CAD build for the part. Positions are in the model's coordinates, mm. Coordinates: 2 decimals unless noted, no trailing zeros. Loops run counter-clockwise (first coordinate to the right, second up) from the corner with the lowest first, then second, coordinate; pieces in that order, holes last. Notation, with made-up numbers: (28.5, -11.75) -> (60.5, -11.75) arc R7 ccw to (60.5, -6.75) -> close; hole circle Ø5 at (9.25, 23.25). An arc over 180 degrees is marked (long way). Return JSON: item names as keys, results as strings. Group by question number.
(1) Saw through at A-A on x = 20.25. Write the cut outline in (y, z) (3 decimals).
(2) Flat gauge pins, fed straight in: pin 1 Ø10 at (x, z) = (17.5, 0.5) entering from -Y; pin 2 Ø2 at (x, z) = (3.5, -2.5) entering from -Y. Where does each tip first touch, or does it go through?
(3) Probe L1, parallel to Z at x = 19.75, y = 64 (3 decimals); L2, parallel to Z at x = 23.75, y = 63; L3, parallel to Y at x = 11, z = 11.5. List the from-to ranges inside material, lowest first.
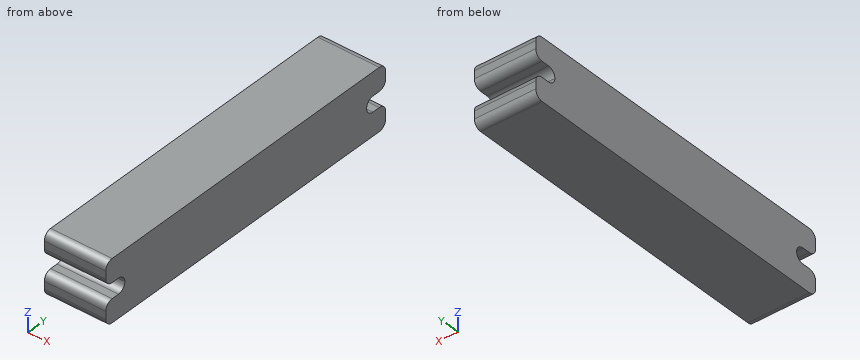
```python
from build123d import *

# Parameters (mm, degrees)
F1_DEPTH = 25.4


with BuildPart() as f1:
    # F0 (on Right) → F1 (new body)
    with BuildSketch(Plane.YZ):
        with BuildLine():
            Line((66.675, 12.7), (-66.675, 12.7))
            ThreePointArc((-66.675, 12.7), (-68.920064, 11.770064), (-69.85, 9.525))
            Line((-69.85, 9.525), (-69.85, 6.35))
            ThreePointArc((-69.85, 6.35), (-68.920064, 4.104936), (-66.675, 3.175))
            Line((-66.675, 3.175), (-63.5, 3.175))
            ThreePointArc((-63.5, 3.175), (-61.254936, 2.245064), (-60.325, 0))
            ThreePointArc((-60.325, 0), (-61.254936, -2.245064), (-63.5, -3.175))
            Line((-63.5, -3.175), (-66.675, -3.175))
            ThreePointArc((-66.675, -3.175), (-68.920064, -4.104936), (-69.85, -6.35))
            Line((-69.85, -6.35), (-69.85, -9.525))
            ThreePointArc((-69.85, -9.525), (-68.920064, -11.770064), (-66.675, -12.7))
            Line((-66.675, -12.7), (66.675, -12.7))
            ThreePointArc((66.675, -12.7), (68.920064, -11.770064), (69.85, -9.525))
            Line((69.85, -9.525), (69.85, -6.35))
            ThreePointArc((69.85, -6.35), (68.920064, -4.104936), (66.675, -3.175))
            Line((66.675, -3.175), (63.5, -3.175))
            ThreePointArc((63.5, -3.175), (61.254936, -2.245064), (60.325, 0))
            ThreePointArc((60.325, 0), (61.254936, 2.245064), (63.5, 3.175))
            Line((63.5, 3.175), (66.675, 3.175))
            ThreePointArc((66.675, 3.175), (68.920064, 4.104936), (69.85, 6.35))
            Line((69.85, 6.35), (69.85, 9.525))
            ThreePointArc((69.85, 9.525), (68.920064, 11.770064), (66.675, 12.7))
        make_face()
    extrude(amount=F1_DEPTH)


solid = f1.part
```
Geometry results:
{
 "1": {"outline": "(-69.85, -9.525) arc R3.175 ccw to (-66.675, -12.7) -> (66.675, -12.7) arc R3.175 ccw to (69.85, -9.525) -> (69.85, -6.35) arc R3.175 ccw to (66.675, -3.175) -> (63.5, -3.175) arc R3.175 cw to (63.5, 3.175) -> (66.675, 3.175) arc R3.175 ccw to (69.85, 6.35) -> (69.85, 9.525) arc R3.175 ccw to (66.675, 12.7) -> (-66.675, 12.7) arc R3.175 ccw to (-69.85, 9.525) -> (-69.85, 6.35) arc R3.175 ccw to (-66.675, 3.175) -> (-63.5, 3.175) arc R3.175 cw to (-63.5, -3.175) -> (-66.675, -3.175) arc R3.175 ccw to (-69.85, -6.35) -> close"},
 "2": {"pin 1": "y = -69.73", "pin 2": "y = -68.07"},
 "3": {"L1": "-12.7 to -3.175, 3.175 to 12.7", "L2": "-12.7 to -3.14, 3.14 to 12.7", "L3": "-69.16 to 69.16"}
}
